Geometry check sheet. Reference: the model listing, model coordinates, mm. A direction names the side the tool comes from. Coordinates: 2 decimals unless noted, no trailing zeros. Loops run counter-clockwise (first coordinate to the right, second up) from the corner with the lowest first, then second, coordinate; pieces in that order, holes last. Notation, with made-up numbers: (19, 73.5) -> (24, 73.5) arc R9 ccw to (24, 83.5) -> close; hole circle Ø8 at (31.25, 58.25). An arc over 180 degrees is marked (long way). Answer as a JSON object with one key per item and string values.
from build123d import *

# Parameters (mm, degrees)
BOSS_EXTRUDE1_DEPTH      = 350
F_3_0_3_DIAMETER_HOLE1_D = 3
F_3_0_3_DIAMETER_HOLE2_D = 3
SKETCH6_R                = 1.5
CUT_EXTRUDE1_DEPTH       = 351.713558335


with BuildPart() as part:
    # Sketch1 → Boss-Extrude1 (new body)
    with BuildSketch(Plane(origin=(0, 0, 0), x_dir=(1, 0, 0), z_dir=(0, 1, 0))):
        Polygon((0, 0), (0, 10), (2, 10), (2, 2), (20, 2), (20, 0), align=None)
    extrude(amount=BOSS_EXTRUDE1_DEPTH)

    # Ø3.0 (3) Diameter Hole1 (through all)
    with Locations(Plane(origin=(2, -11.407632793, -188.67995168), x_dir=(0, 0, -1), z_dir=(1, 0, 0))):
        with Locations((-182.67995168, 17.407632793), (-182.67995168, 31.407632793)):
            Hole(F_3_0_3_DIAMETER_HOLE1_D / 2)

    # Ø3.0 (3) Diameter Hole2 (through all)
    with Locations(Plane(origin=(2, -11.407632793, -188.67995168), x_dir=(0, 0, -1), z_dir=(1, 0, 0))):
        with Locations((-182.67995168, 355.407632793), (-182.67995168, 341.407632793)):
            Hole(F_3_0_3_DIAMETER_HOLE2_D / 2)

    # Sketch6 → Cut-Extrude1 (cut, through all)
    with BuildSketch(Plane.XY):
        with Locations((12.999999986, 290)):
            Circle(SKETCH6_R)
        with Locations((12.999999986, 270)):
            Circle(SKETCH6_R)
        with Locations((12.999999986, 250)):
            Circle(SKETCH6_R)
        with Locations((12.999999986, 230)):
            Circle(SKETCH6_R)
        with Locations((12.999999986, 210)):
            Circle(SKETCH6_R)
        with Locations((12.999999986, 190)):
            Circle(SKETCH6_R)
        with Locations((12.999999986, 170)):
            Circle(SKETCH6_R)
        with Locations((12.999999986, 150)):
            Circle(SKETCH6_R)
        with Locations((12.999999986, 130)):
            Circle(SKETCH6_R)
        with Locations((12.999999986, 110)):
            Circle(SKETCH6_R)
        with Locations((12.999999986, 90)):
            Circle(SKETCH6_R)
        with Locations((12.999999986, 70)):
            Circle(SKETCH6_R)
        with Locations((12.999999986, 50)):
            Circle(SKETCH6_R)
    extrude(amount=-CUT_EXTRUDE1_DEPTH, mode=Mode.SUBTRACT)


solid = part.part
1. Section check C-C, the plane x = 6. Record the boundary of the cut face in (y, z), then the cut area to 3 significant figures.
Evaluation:
{"outline": "(0, -2) -> (350, -2) -> (350, 0) -> (0, 0) -> close", "area": "700 mm^2"}
2. Tool access check on faces 1 (the face through (2, 173, -6)), 2 (the face through (7.1, 0, -1.7)). Record the directions out of +Z, -Z, +X, -X, +Y, -Y that give a thin tool (end or side, any length) a straight path to the whole face; none if there is none.
Evaluation:
{"face 1": "-Z, +X, +Y, -Y", "face 2": "+Z, -Z, +X, -X, -Y"}
3. Section check B-B, the plane y = 223.5. Record the boundary of the cut face in (x, z), then the cut area to 3 significant figures.
Evaluation:
{"outline": "(0, -10) -> (2, -10) -> (2, -2) -> (20, -2) -> (20, 0) -> (0, 0) -> close", "area": "56.0 mm^2"}
4. Depth check by flat-ended pin: P1, Ø4, axis at x = 12, y = 58.5, coming from the -Z side; P2, Ø2.5, axis at y = 255.5, z = -7, coming from the +X side. Enter the tip coordinate at first touch or a pass-through.
Evaluation:
{"P1": "stops at z = -2", "P2": "stops at x = 2"}
5. Section check A-A, the plane z = -6. Record the boundary of the cut face in (x, y).
Evaluation:
{"outline": "(0, 0) -> (2, 0) -> (2, 4.5) -> (0, 4.5) -> close; (0, 7.5) -> (2, 7.5) -> (2, 18.5) -> (0, 18.5) -> close; (0, 21.5) -> (2, 21.5) -> (2, 328.5) -> (0, 328.5) -> close; (0, 331.5) -> (2, 331.5) -> (2, 342.5) -> (0, 342.5) -> close; (0, 345.5) -> (2, 345.5) -> (2, 350) -> (0, 350) -> close"}
6. Thickness scan on probe 1 along Y at (x, z) = (0.6, -6); probe 2 along X at (y, z) = (90, -0.7); probe 3 along Z at (x, y) = (19, 175). Record the ranges inside material, lowest first. Write a range as from..to.
Evaluation:
{"probe 1": "y = 0..4.5, 7.5..18.5, 21.5..328.5, 331.5..342.5, 345.5..350", "probe 2": "x = 0..11.5, 14.5..20", "probe 3": "z = -2..0"}
